Check sheet for the modelled part. Datum: model origin and axes. Units: mm. A direction names the side the tool comes from. Round coordinates to 2 decimals unless told otherwise and drop trailing zeros. Loops run counter-clockwise (first coordinate to the right, second up) from the corner with the lowest first, then second, coordinate; pieces in that order, holes last. Notation, with made-up numbers: (34, 40) - (52, 40) arc R18 cw to (52, 68) - close; hole circle Ø9 at (-34, 86). An arc over 180 degrees is marked (long way). Answer in a Markdown table with one row per item. Add a question column.
(1) Gauge pin test, flat ends, axial feed: pin 1 (1.5 mm diameter, centred on x = -0.5, z = 0.5, fed in from -Y); pin 2 (2 mm diameter, centred on y = -3, z = 7.5, fed in from -X); pin 3 (1 mm diameter, centred on y = -5, z = 3.5, fed in from +X). Record the tip position at first contact, or that the pin passes through.
(2) Cross-section at A-A on x = 0. Enter the section's corners in (y, z), then the cut area to 3 significant figures.
(3) Cross-section at B-B on y = -3. Enter the section's corners in (x, z), then the cut area to 3 significant figures.
(4) Cross-section at C-C on z = 0. Enter the section's corners in (x, y), then the cut area to 3 significant figures.
(5) Mould release check, pull along Z, two halves, no side actions. Record for faces 3 (the cylindrical face through (3.233, -4.739, -1.341)), 4 (the flat face through (2, -7, -2)), 5 (the cylindrical face through (-0.54, -4.74, -2.44)): +Z half, -Z half, draft (parallel to the pull), parting line (faces both ways), or undercut.
(6) Cross-section at D-D on z = 5.75. Enter the section's corners in (x, y).
(7) Access from +Z, -Z, +X, -X, +Y, -Y to the whole of each face (thin tool, end or side, straight path). Record for faces 1 (the flat face through (0, 0, 0)), 2 (the flat face through (0, -2.54, 0)).
(8) Thickness scan on line 1 along Z through (x, y) = (0, -5.25); line 2 along Y through (x, z) = (-3.5, 3.5). Record the ranges inside material, lowest first.
from build123d import *

# Parameters (mm, degrees)
F0_R     = 3.5
F0_R_2   = 2.5
F1_DEPTH = 7
F2_R     = 11
F3_DEPTH = 2.54


with BuildPart() as f1:
    # F0 (on Front) → F1 (new body)
    with BuildSketch(Plane.XZ):
        Circle(F0_R)
        Circle(F0_R_2, mode=Mode.SUBTRACT)
    extrude(amount=F1_DEPTH)

    # F2 (on Front) → F3 (join)
    with BuildSketch(Plane.XZ):
        Circle(F2_R)
    extrude(amount=F3_DEPTH)


solid = f1.part
Answers:
| question | item | result |
|---|---|---|
| 1 | pin 1 | stops at y = -2.54 |
| 1 | pin 2 | stops at x = -8.79 |
| 1 | pin 3 | stops at x = 1.8 |
| 2 | outline | (-7, -3.5) - (-2.54, -3.5) - (-2.54, -11) - (0, -11) - (0, 11) - (-2.54, 11) - (-2.54, 3.5) - (-7, 3.5) - (-7, 2.5) - (-2.54, 2.5) - (-2.54, -2.5) - (-7, -2.5) - close |
| 2 | area | 64.8 mm^2 |
| 3 | outline | circle Ø7 at (0, 0); hole circle Ø5 at (0, 0) |
| 3 | area | 18.8 mm^2 |
| 4 | outline | (-11, -2.54) - (-3.5, -2.54) - (-3.5, -7) - (-2.5, -7) - (-2.5, -2.54) - (2.5, -2.54) - (2.5, -7) - (3.5, -7) - (3.5, -2.54) - (11, -2.54) - (11, 0) - (-11, 0) - close |
| 4 | area | 64.8 mm^2 |
| 5 | face 3 | parting line |
| 5 | face 4 | draft |
| 5 | face 5 | undercut |
| 6 | outline | (-9.38, -2.54) - (9.38, -2.54) - (9.38, 0) - (-9.38, 0) - close |
| 7 | face 1 | +Z, -Z, +X, -X, +Y |
| 7 | face 2 | -Y |
| 8 | line 1 | z = -3.5 to -2.5, 2.5 to 3.5 |
| 8 | line 2 | y = -2.54 to 0 |
